Read the model definition and answer for the solid it produces. Units are mm, in the model's axes. Coordinates: 2 decimals unless noted, no trailing zeros. Loops run counter-clockwise (first coordinate to the right, second up) from the corner with the lowest first, then second, coordinate; pieces in that order, holes last. Notation, with made-up numbers: (59.5, -10.5) - (111.5, -10.5) arc R23 cw to (111.5, 4.5) - close; hole circle Ø3 at (51, -21). An arc over 180 degrees is marked (long way). Use CSV: the item, a comma, the result in double quotes.
```python
from build123d import *

# Parameters (mm, degrees)
BOSS_EXTRUDE1_DEPTH = 4.50088
CUT_EXTRUDE1_DEPTH  = 4.50088
CIRPATTERN1_COUNT   = 4
CUT_EXTRUDE3_DEPTH  = 5.50088
CIRPATTERN2_COUNT   = 4
SKETCH6_R           = 3.175
CUT_EXTRUDE4_DEPTH  = 5.50088
CIRPATTERN3_COUNT   = 4
SKETCH9_R           = 2.54
CUT_EXTRUDE5_DEPTH  = 5.50088
CIRPATTERN4_COUNT   = 4


with BuildPart() as part:
    # Sketch1 → Boss-Extrude1 (new body)
    with BuildSketch(Plane(origin=(0, 0, 0), x_dir=(1, 0, 0), z_dir=(0, 1, 0))):
        with BuildLine():
            Line((-66.675, 0), (-50.8, 0))
            Line((-50.8, 0), (-50.8, 16.51))
            Line((-50.8, 16.51), (-56.248410053, 16.51))
            ThreePointArc((-56.248410053, 16.51), (-58.837856989, 17.84777667), (-59.245192619, 20.733770352))
            ThreePointArc((-59.245192619, 20.733770352), (-44.384017853, 44.384017853), (-20.733770352, 59.245192619))
            ThreePointArc((-20.733770352, 59.245192619), (-17.84777667, 58.837856989), (-16.51, 56.248410053))
            Line((-16.51, 56.248410053), (-16.51, 50.8))
            Line((-16.51, 50.8), (0, 50.8))
            Line((0, 50.8), (0, 66.675))
            ThreePointArc((0, 66.675), (-47.146344636, 47.146344636), (-66.675, 0))
        make_face()
    boss_extrude1 = extrude(amount=BOSS_EXTRUDE1_DEPTH)

    # Sketch2 → Cut-Extrude1 (cut)
    with BuildSketch(Plane(origin=(0, 4.50088, 0), x_dir=(1, 0, 0), z_dir=(0, 1, 0))):
        Polygon((-63.024379444, 7.772955042), (-57.963710378, 7.330203869), (-58.355987918, 2.846451076), (-63.416656984, 3.28920225), align=None)
        Polygon((-7.330203869, 57.963710378), (-5.088327473, 58.159849148), (-5.531078646, 63.220518214), (-7.772955042, 63.024379444), align=None)
        Polygon((-5.531078646, 63.220518214), (-5.088327473, 58.159849148), (-2.846451076, 58.355987918), (-3.28920225, 63.416656984), align=None)
    cut_extrude1 = extrude(amount=-CUT_EXTRUDE1_DEPTH, mode=Mode.SUBTRACT)

    # CirPattern1: Boss-Extrude1, Cut-Extrude1 ×4 about axis
    cirpattern1_axis = Axis((0, 0, 0), (0, 1, 0))
    for i in range(1, CIRPATTERN1_COUNT):
        add(boss_extrude1.rotate(cirpattern1_axis, i * 360 / CIRPATTERN1_COUNT))
        add(cut_extrude1.rotate(cirpattern1_axis, i * 360 / CIRPATTERN1_COUNT), mode=Mode.SUBTRACT)

    # Sketch5 → Cut-Extrude3 (cut, through all)
    with BuildSketch(Plane(origin=(0, 4.50088, 0), x_dir=(1, 0, 0), z_dir=(0, 1, 0))):
        with BuildLine():
            Line((-2.54, 50.8), (2.54, 50.8))
            ThreePointArc((2.54, 50.8), (0, 53.34), (-2.54, 50.8))
        make_face()
    cut_extrude3 = extrude(amount=-CUT_EXTRUDE3_DEPTH, mode=Mode.SUBTRACT)

    # CirPattern2: Cut-Extrude3 ×4 about axis
    cirpattern2_axis = Axis((0, 0, 0), (0, 1, 0))
    for i in range(1, CIRPATTERN2_COUNT):
        add(cut_extrude3.rotate(cirpattern2_axis, i * 360 / CIRPATTERN2_COUNT), mode=Mode.SUBTRACT)

    # Sketch6 → Cut-Extrude4 (cut, through all)
    with BuildSketch(Plane(origin=(0, 4.50088, 0), x_dir=(1, 0, 0), z_dir=(0, 1, 0))):
        with Locations((-56.03313088, -11.43)):
            Circle(SKETCH6_R)
    cut_extrude4 = extrude(amount=-CUT_EXTRUDE4_DEPTH, mode=Mode.SUBTRACT)

    # CirPattern3: Cut-Extrude4 ×4 about axis
    cirpattern3_axis = Axis((0, 0, 0), (0, 1, 0))
    for i in range(1, CIRPATTERN3_COUNT):
        add(cut_extrude4.rotate(cirpattern3_axis, i * 360 / CIRPATTERN3_COUNT), mode=Mode.SUBTRACT)

    # Sketch9 → Cut-Extrude5 (cut, through all)
    with BuildSketch(Plane(origin=(0, 4.50088, 0), x_dir=(1, 0, 0), z_dir=(0, 1, 0))):
        with Locations((11.43, 56.03313088)):
            Circle(SKETCH9_R)
    cut_extrude5 = extrude(amount=-CUT_EXTRUDE5_DEPTH, mode=Mode.SUBTRACT)

    # CirPattern4: Cut-Extrude5 ×4 about axis
    cirpattern4_axis = Axis((0, 0, 0), (0, 1, 0))
    for i in range(1, CIRPATTERN4_COUNT):
        add(cut_extrude5.rotate(cirpattern4_axis, i * 360 / CIRPATTERN4_COUNT), mode=Mode.SUBTRACT)


solid = part.part
```
Q1. The part is cut by section B-B on z = -11.43. Determine the outline of the cut face in (x, y), and give its area (3 significant figures).
Reported:
outline,"(-65.69, 0) - (-58.57, 0) - (-58.57, 4.5) - (-65.69, 4.5) - close; (-53.49, 0) - (-50.8, 0) - (-50.8, 4.5) - (-53.49, 4.5) - close; (50.8, 0) - (52.86, 0) - (52.86, 4.5) - (50.8, 4.5) - close; (59.21, 0) - (65.69, 0) - (65.69, 4.5) - (59.21, 4.5) - close"
area,"82.6 mm²"
Q2. The part is cut by section D-D on y = 2.3. Give the number of separate pieces and of enclosed holes in the cut face, and give its area (3 significant figures).
Reported:
separate pieces,"1"
enclosed holes,"17"
area,"2,680 mm²"
Q3. For a pull along Z with two mould halves and no side action, classify faces 1 (the face through (58.86, 2.22, -17.88)), 2 (the face through (50.8, 2, -10)), 3 (the face through (-54, 4.501, 0)) as +Z half, -Z half, draft (parallel to the pull), parting line (faces both ways), or undercut.
Reported:
face 1,"undercut"
face 2,"undercut"
face 3,"draft"
Q4. The part is cut by section A-A on x = 44.5. Determine the outline of the cut face in (y, z), and give its area (3 significant figures).
Reported:
outline,"(0, -49.65) - (4.5, -49.65) - (4.5, -44.27) - (0, -44.27) - close; (0, 44.27) - (4.5, 44.27) - (4.5, 49.65) - (0, 49.65) - close"
area,"48.5 mm²"
Q5. Find the intervals of material crossed by probe 1 along Z at (x, y) = (12, 2.5); probe 2 along Z at (x, y) = (-57, 2); probe 3 along X at (y, z) = (0.75, -12.5), in increasing order. Write a range as [from, to].
Reported:
probe 1,"z = [-65.59, -58.51], [-53.56, -50.8], [50.8, 52.91], [59.16, 65.59]"
probe 2,"z = [-34.59, -26.28], [-16.6, -13.78], [-9.08, 8.41], [14.45, 16.6], [26.28, 34.59]"
probe 3,"x = [-65.49, -58.34], [-53.73, -50.8], [50.8, 53.04], [59.02, 65.49]"
Q6. Given P1, Ø2.5, axis at x = 52.5, y = 1.5, coming from the -Z side; P2, Ø2.5, axis at x = -7.5, y = 3, coming from the -Z side; P3, Ø2.5, axis at x = -53, y = 1.5, coming from the -Z side, each flat-ended and moving along its own axis, determine where each tip first touches the part or whether it passes through.
Reported:
P1,"stops at z = -42.65"
P2,"stops at z = -66.38"
P3,"stops at z = -42.04"
Q7. The part is cut by section C-C on x = 11.43. Determine the outline of the cut face in (y, z), and give its area (3 significant figures).
Reported:
outline,"(0, -65.69) - (4.5, -65.69) - (4.5, -58.57) - (0, -58.57) - close; (0, -53.49) - (4.5, -53.49) - (4.5, -50.8) - (0, -50.8) - close; (0, 50.8) - (4.5, 50.8) - (4.5, 52.86) - (0, 52.86) - close; (0, 59.21) - (4.5, 59.21) - (4.5, 65.69) - (0, 65.69) - close"
area,"82.6 mm²"
